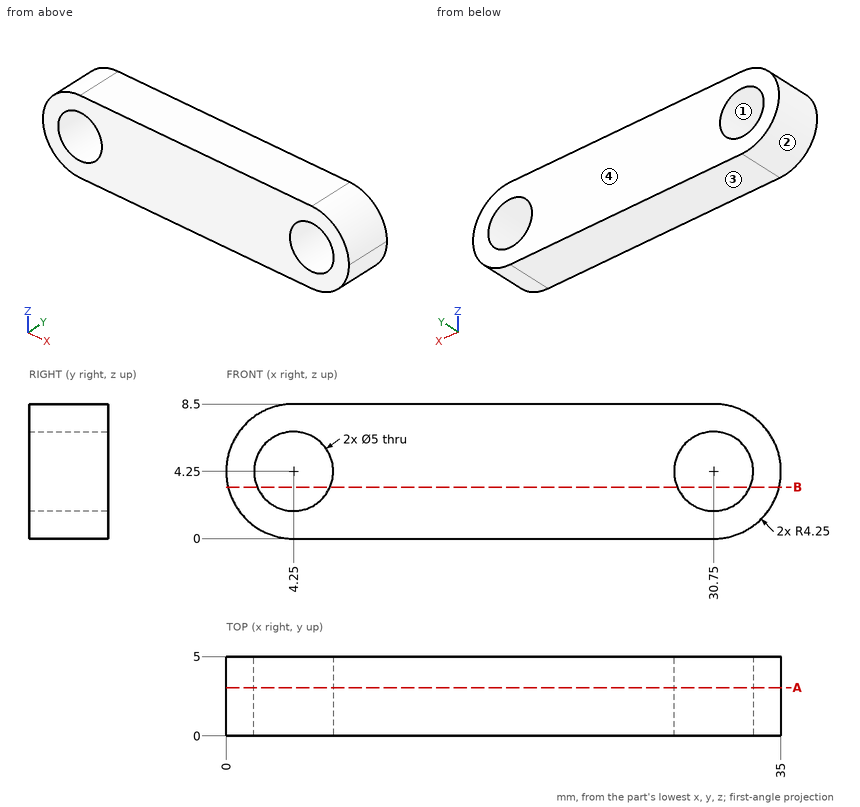
Geometry check sheet. Reference: drawing and pictorial views, mm from the part's lowest x, y, z. Give positions to 0.01 mm unless a question says otherwise; leave off trailing zeros. Order: outer loops, then holes, each group sorted by start corner. A loop starts at its lowest first (then second) coordinate and runs counter-clockwise, first axis right, second up. Notation, with made-up numbers: (-6, 83) - (46, 83) arc R12 cw to (46, 95) - close; hole circle Ø10 at (61.5, 32). An arc over 180 degrees is marked (long way). Use one line per item in the form item = value.
1) Depth check by flat-ended pin: pin 1 Ø2 at (y, z) = (1.5, 3) entering from +X. Enter the tip coordinate at first touch or a pass-through.
Working result:
pin_1 = 34.99
2) Sectioned sample at B-B (z = 3.25). Record the boundary of the cut face in (x, y), and give its area (3 significant figures).
Working result:
outline = (0.12, 0) - (1.96, 0) - (1.96, 5) - (0.12, 5) - close; (6.54, 0) - (28.46, 0) - (28.46, 5) - (6.54, 5) - close; (33.04, 0) - (34.88, 0) - (34.88, 5) - (33.04, 5) - close
area = 128 mm^2
3) Draft check along Z on the marked faces 1, 2, 3 and 4. Enter one of: released by +Z, released by -Z, zero draft, split by the parting line, or undercut.
Working result:
face_1 = undercut
face_2 = split by the parting line
face_3 = released by -Z
face_4 = zero draft
4) Material ranges on probe 1 along Z at (x, y) = (4.25, 3.5); probe 2 along X at (y, z) = (2.45, 5); probe 3 along X at (y, z) = (0.8, 3), recorded low to high. Write a range as from..to.
Working result:
probe_1 = 0..1.75, 6.75..8.5
probe_2 = 0.07..1.87, 6.63..28.37, 33.13..34.93
probe_3 = 0.19..2.08, 6.42..28.58, 32.92..34.81
5) Sectioned sample at A-A (y = 3.05). Record the boundary of the cut face in (x, z), and give its area (3 significant figures).
Working result:
outline = (4.25, 0) - (30.75, 0) arc R4.25 ccw to (35, 4.25) arc R4.25 ccw to (30.75, 8.5) - (4.25, 8.5) arc R4.25 ccw to start; hole circle Ø5 at (4.25, 4.25); hole circle Ø5 at (30.75, 4.25)
area = 243 mm^2
